```python
from build123d import *

# Parameters (mm, degrees)
CROQUIS1_R              = 9.75
SALIENTE_EXTRUIR1_DEPTH = 6
CROQUIS2_R              = 1.5
CORTAR_EXTRUIR1_DEPTH   = 6
CROQUIS3_R              = 3
CORTAR_EXTRUIR2_DEPTH   = 6
REDONDEO1_R             = 1


with BuildPart() as part:
    # Croquis1 → Saliente-Extruir1 (new body)
    with BuildSketch(Plane(origin=(0, 0, 0), x_dir=(1, 0, 0), z_dir=(0, 1, 0))):
        with BuildLine():
            ThreePointArc((12.5, 0), (0, 12.5), (-12.5, 0))
            Line((-12.5, 0), (-12.5, -16))
            ThreePointArc((-12.5, -16), (-13.085786438, -17.414213562), (-14.5, -18))
            Line((-14.5, -18), (-20.5, -18))
            Line((-20.5, -18), (-20.5, -21))
            Line((-20.5, -21), (-5.5, -21))
            Line((-5.5, -21), (-5.5, -31))
            Line((-5.5, -31), (5.5, -31))
            Line((5.5, -31), (5.5, -21))
            Line((5.5, -21), (20.5, -21))
            Line((20.5, -21), (20.5, -18))
            Line((20.5, -18), (14.5, -18))
            ThreePointArc((14.5, -18), (13.085786438, -17.414213562), (12.5, -16))
            Line((12.5, -16), (12.5, 0))
        make_face()
        Circle(CROQUIS1_R, mode=Mode.SUBTRACT)
    extrude(amount=SALIENTE_EXTRUIR1_DEPTH)

    # Croquis2 → Cortar-Extruir1 (cut)
    with BuildSketch(Plane.XY.offset(21)):
        with Locations((-16.5, 3)):
            Circle(CROQUIS2_R)
        with Locations((16.5, 3)):
            Circle(CROQUIS2_R)
    extrude(amount=-CORTAR_EXTRUIR1_DEPTH, mode=Mode.SUBTRACT)

    # Croquis3 → Cortar-Extruir2 (cut)
    with BuildSketch(Plane(origin=(0, 0, 18), x_dir=(-1, 0, 0), z_dir=(0, 0, -1))):
        with Locations((-16.5, 3)):
            Circle(CROQUIS3_R)
        with Locations((16.5, 3)):
            Circle(CROQUIS3_R)
    extrude(amount=CORTAR_EXTRUIR2_DEPTH, mode=Mode.SUBTRACT)

    # Redondeo1
    redondeo1_edges = [part.edges().sort_by_distance(p)[0] for p in [
        (5.5, 3, 31),
        (-5.5, 3, 31),
        (0, 6, 31),
        (0, 0, 31),
    ]]
    fillet(redondeo1_edges, radius=REDONDEO1_R)


solid = part.part
```
Geometry: final body of the model. Coordinates: model frame, mm. A direction names the side the tool comes from. Coordinates: 2 decimals unless noted, no trailing zeros. Write each loop counter-clockwise with the first axis right and the second up, starting at its lowest first coordinate (ties: lowest second). Pieces come first, ordered by that corner, then holes. Notation, with made-up numbers: M -23.5,-21.5 L 2.5,-21.5 A16 cw 2.5,7.5 Z; hole C -8.5,87.25 d11. An arc over 180 degrees is marked long. Answer as CSV lines item,"result". Start each with the question number.
Q1. Reachability of faces 5 (the flat face through (-12.5, 3, 8)), 6 (the flat face through (-5.5, 3, 25)), 7 (the flat face through (-20.5, 3, 19)) from +Z, -Z, +X, -X, +Y, -Y: full face, straight path, thin tool, end or side. Return the list, or none.
Q2. Mould query, pull axis Y, two halves, no side actions, for faces 1 (the cylindrical face through (15, 3, 20)), 2 (the flat face through (-13, 3, 21)), 3 (the cylindrical face through (-18, 3, 20)), 4 (the cylindrical face through (0.077, 0.301, 30.715)). Classes: released by +Y, released by -Y, zero draft, split by the parting line, or undercut.
Q3. Cut plane D-D on z = -6. Return the cut outline in (x, y).
Q4. Cut plane B-B on x = 0. Return the cut outline in (y, z).
Q5. Cut plane C-C on z = 19.5. Return the cut outline in (x, y), then the cut area to 3 significant figures.
Q6. Line query: line 1 (Z direction, x = 0, y = 2.8); line 2 (X direction, y = 1.75, z = 19); line 3 (Y direction, x = 16.5, z = 20.1). Output: solid intervals per line, ascending. Write a range as from..to.
Q7. Cut plane A-A on y = 3. Return the cut outline in (x, z).
Q8. Pin query (flat end, axial travel): P1, Ø1, axis at x = -2.5, y = 2, coming from the -Z side; P2, Ø1.8, axis at x = -11.5, y = 4, coming from the +Z side; P3, Ø1.8, axis at x = 15.5, y = 2.5, coming from the -Z side; P4, Ø1.8, axis at x = -16.5, y = 3, coming from the -Z side. Return the tip coordinate at first contact, or that it passes through.
Findings below:
1,face 5,"-Z, -X, +Y, -Y"
1,face 6,"+Z, -X, +Y, -Y"
1,face 7,"+Z, -Z, -X, +Y, -Y"
2,face 1,"undercut"
2,face 2,"zero draft"
2,face 3,"undercut"
2,face 4,"released by -Y"
3,outline,"M -10.97,0 L -7.69,0 L -7.69,6 L -10.97,6 Z; M 7.69,0 L 10.97,0 L 10.97,6 L 7.69,6 Z"
4,outline,"M 0,-12.5 L 6,-12.5 L 6,-9.75 L 0,-9.75 Z; M 0,9.75 L 6,9.75 L 6,30 A1 ccw 5,31 L 1,31 A1 ccw 0,30 Z"
5,outline,"M -20.5,0 L 20.5,0 L 20.5,6 L -20.5,6 Z; hole C -16.5,3 d3; hole C 16.5,3 d3"
5,area,"232 mm2"
6,line 1,"z = -12.5..-9.75, 9.75..31"
6,line 2,"x = -20.5..-17.33, -15.67..15.67, 17.33..20.5"
6,line 3,"y = 0..1.5, 4.5..6"
7,outline,"M -20.5,18 L -18,18 L -18,21 L -20.5,21 Z; M -15,18 L -13.5,18 L -13.5,17.73 A2 cw -12.5,16 L -12.5,0 A12.5 ccw 12.5,0 L 12.5,16 A2 cw 13.5,17.73 L 13.5,18 L 15,18 L 15,21 L 5.5,21 L 5.5,30 A1 ccw 4.5,31 L -4.5,31 A1 ccw -5.5,30 L -5.5,21 L -15,21 Z; M 18,18 L 20.5,18 L 20.5,21 L 18,21 Z; hole C 0,0 d19.5"
8,P1,"stops at z = -12.34"
8,P2,"stops at z = 21"
8,P3,"stops at z = 18"
8,P4,"passes through"
